Here's how the part is built. I have some questions about the finished solid (model axes, mm). Face numbers are marked on the shaded views. Round coordinates to 2 decimals unless told otherwise and drop trailing zeros. Order: outer loops, then holes, each group sorted by start corner. A loop starts at its lowest first (then second) coordinate and runs counter-clockwise, first axis right, second up. Notation, with made-up numbers: (-25, 5) -> (-17, 5) arc R9 cw to (-17, 17) -> close; hole circle Ø3 at (-7.75, -28). An arc over 180 degrees is marked (long way). One line per item, written item: value.
```python
from build123d import *

# Parameters (mm, degrees)
SKETCH1_R           = 20
SKETCH1_R_2         = 2.75
BOSS_EXTRUDE1_DEPTH = 2.5
CUT_EXTRUDE3_DEPTH  = 2.5
SKETCH4_R           = 1.25
CUT_EXTRUDE4_DEPTH  = 5
SKETCH2_R           = 3
SKETCH2_R_2         = 2.75
BOSS_EXTRUDE2_DEPTH = 15


with BuildPart() as part:
    # Sketch1 → Boss-Extrude1 (new body)
    with BuildSketch(Plane(origin=(0, 0, 0), x_dir=(1, 0, 0), z_dir=(0, 1, 0))):
        Circle(SKETCH1_R)
        Circle(SKETCH1_R_2, mode=Mode.SUBTRACT)
    extrude(amount=BOSS_EXTRUDE1_DEPTH)

    # Sketch3 → Cut-Extrude3 (cut)
    with BuildSketch(Plane.XZ):
        Polygon((-5.161329605, 1.721273866), (-8.071331697, 3.318997608), (-10.910002092, 1.597723742), (-10.838670395, -1.721273866), (-7.928668303, -3.318997608), (-5.089997908, -1.597723742), align=None)
        Polygon((5.161329605, -1.721273866), (8.071331697, -3.318997608), (10.910002092, -1.597723742), (10.838670395, 1.721273866), (7.928668303, 3.318997608), (5.089997908, 1.597723742), align=None)
    extrude(amount=-CUT_EXTRUDE3_DEPTH, mode=Mode.SUBTRACT)

    # Sketch4 → Cut-Extrude4 (cut)
    with BuildSketch(Plane(origin=(0, 2.5, 0), x_dir=(1, 0, 0), z_dir=(0, 1, 0))):
        with Locations((0, 17)):
            Circle(SKETCH4_R)
        with Locations((0, 20)):
            Circle(SKETCH4_R)
    extrude(amount=-CUT_EXTRUDE4_DEPTH, mode=Mode.SUBTRACT)

    # Sketch2 → Boss-Extrude2 (add)
    with BuildSketch(Plane(origin=(0, 2.5, 0), x_dir=(1, 0, 0), z_dir=(0, 1, 0))):
        Circle(SKETCH2_R)
        Circle(SKETCH2_R_2, mode=Mode.SUBTRACT)
    extrude(amount=BOSS_EXTRUDE2_DEPTH)

    # Mirror7: part across plane


with BuildPart() as part_1:
    add(part.part)
    add(part.part.mirror(Plane.ZX.offset(17.5)))


solid = part_1.part
```
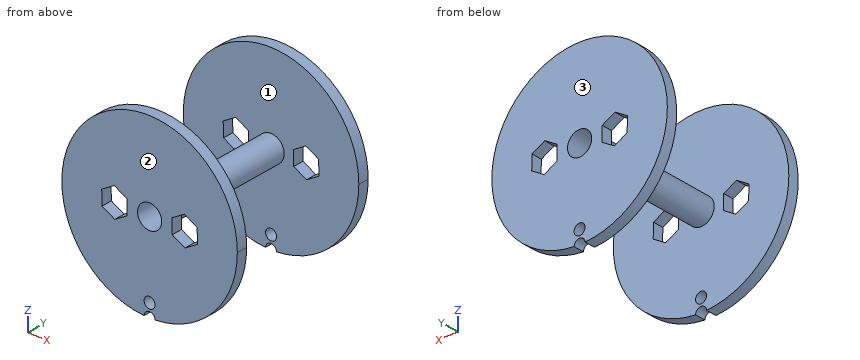
Q1. I want a section at D-D on y = 19. Write out the boundary of the cut face in (x, z).
Answers:
outline: circle Ø6 at (0, 0); hole circle Ø5.5 at (0, 0)
Q2. I want a section at A-A on x = 0. Write out the boundary of the cut face in (y, z).
Answers:
outline: (0, -18.75) -> (2.5, -18.75) -> (2.5, -18.25) -> (0, -18.25) -> close; (0, -15.75) -> (2.5, -15.75) -> (2.5, -3) -> (32.5, -3) -> (32.5, -15.75) -> (35, -15.75) -> (35, -2.75) -> (0, -2.75) -> close; (0, 2.75) -> (35, 2.75) -> (35, 20) -> (32.5, 20) -> (32.5, 3) -> (2.5, 3) -> (2.5, 20) -> (0, 20) -> close; (32.5, -18.75) -> (35, -18.75) -> (35, -18.25) -> (32.5, -18.25) -> close
Q3. For P1, Ø12, axis at x = 2.5, y = 22.5, coming from the -Z side; P2, Ø8, axis at x = 1.5, y = 19.5, coming from the +Z side; P3, Ø2, axis at y = 18.5, z = 1.5, coming from the -X side, each with a flat end and sliding along its axis, tell me the tip position at first contact or that it passes through.
Answers:
P1: z = -3
P2: z = 3
P3: x = -2.96
Q4. I want a section at B-B on z = -12. Write out the boundary of the cut face in (x, y), then the cut area to 3 significant figures.
Answers:
outline: (-16, 0) -> (16, 0) -> (16, 2.5) -> (-16, 2.5) -> close; (-16, 32.5) -> (16, 32.5) -> (16, 35) -> (-16, 35) -> close
area: 160 mm2
Q5. If we mould it in two halves opening along Y, with no side actions, what happens to the marked faces 1, 2 and 3? For each: pulls with the +Y half, pulls with the -Y half, needs draft (parallel to the pull), parting line crosses it, or undercut.
Answers:
face 1: undercut
face 2: pulls with the -Y half
face 3: pulls with the +Y half
Q6. I want a section at C-C on x = 13. Write out the boundary of the cut face in (y, z).
Answers:
outline: (0, -15.2) -> (2.5, -15.2) -> (2.5, 15.2) -> (0, 15.2) -> close; (32.5, -15.2) -> (35, -15.2) -> (35, 15.2) -> (32.5, 15.2) -> close
Q7. I need wall thicknesses on line 1 along Z through (x, y) = (0, 1); line 2 along Y through (x, z) = (0.5, 9.5); line 3 along Z through (x, y) = (0, 5). Which ranges of each line are inside material? Lowest first, please.
Answers:
line 1: -18.75 to -18.25, -15.75 to -2.75, 2.75 to 20
line 2: 0 to 2.5, 32.5 to 35
line 3: -3 to -2.75, 2.75 to 3
